Here's the drawing with two shaded views (mm, measured from the low corner). I have some questions. A direction names the side the tool comes from. Coordinates: 2 decimals unless noted, no trailing zeros. Write each loop counter-clockwise with the first axis right and the second up, starting at its lowest first coordinate (ties: lowest second). Pieces come first, ordered by that corner, then holes.
Item 1: For P1, Ø7, axis at x = 21, y = 12, coming from the -Z side; P2, Ø0.6, axis at y = 1, z = 0.5, coming from the -X side; P3, Ø0.6, axis at y = 0.5, z = 0.5, coming from the +X side; P4, Ø4, axis at x = 39, y = 17, coming from the +Z side, each with a flat end and sliding along its axis, tell me the tip position at first contact or that it passes through.
Item 2: I want a section at D-D on z = 0.6. Please give me the cut outline in (x, y).
Item 3: If I drill on probe 1 along Y at (x, z) = (4, 0.8) (1 decimal); probe 2 along X at (y, z) = (16.5, 0.45) (1 decimal); probe 3 along X at (y, z) = (17.5, 1.5) (1 decimal), over which ranges is the centre line in solid material (lowest first)?
Item 4: I want a section at B-B on y = 10.25. Please give me the cut outline in (x, z).
Item 5: I want a section at A-A on x = 39. Please give me the cut outline in (y, z), then the cut area to 3 significant figures.
Item 6: I want a section at C-C on x = 22.5. Please give me the cut outline in (y, z) (1 decimal).
Item 7: Which directions (+Z, -Z, +X, -X, +Y, -Y) give clear straight access to the entire face, cutting with the end or side of a thin tool? Please do the marked faces 1 and 2.
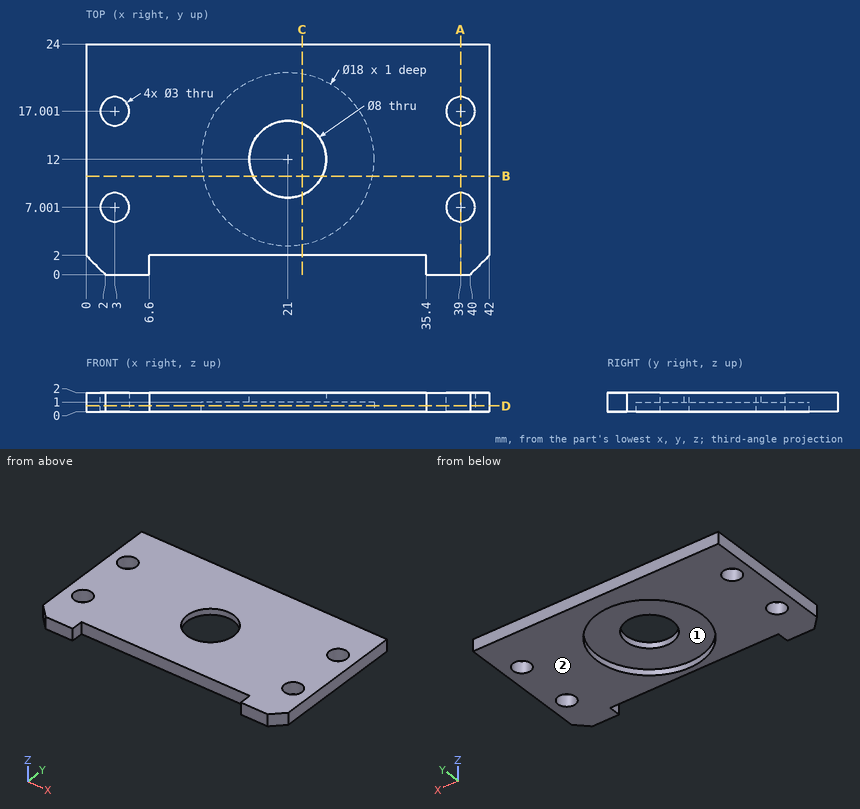
Response values:
1. P1: passes through
1. P2: stops at x = 0.7
1. P3: stops at x = 40.8
1. P4: stops at z = 2
2. outline: (0, 2) - (2, 0) - (6.6, 0) - (6.6, 2) - (35.4, 2) - (35.4, 0) - (40, 0) - (42, 2) - (42, 24) - (0, 24) - close; hole circle Ø3 at (3, 7); hole circle Ø3 at (3, 17); hole circle Ø18 at (21, 12); hole circle Ø3 at (39, 7); hole circle Ø3 at (39, 17)
3. probe 1: y = 0 to 5.9, 8.1 to 15.9, 18.1 to 24
3. probe 2: x = 0 to 1.6, 4.4 to 13.2, 28.8 to 37.6, 40.4 to 42
3. probe 3: x = 0 to 1.6, 4.4 to 37.6, 40.4 to 42
4. outline: (0, 0) - (12.17, 0) - (12.17, 1) - (17.4, 1) - (17.4, 2) - (0, 2) - close; (24.6, 1) - (29.83, 1) - (29.83, 0) - (42, 0) - (42, 2) - (24.6, 2) - close
5. outline: (0, 0) - (5.5, 0) - (5.5, 2) - (0, 2) - close; (8.5, 0) - (15.5, 0) - (15.5, 2) - (8.5, 2) - close; (18.5, 0) - (24, 0) - (24, 2) - (18.5, 2) - close
5. area: 36.0 mm2
6. outline: (2, 0) - (3.1, 0) - (3.1, 1) - (8.3, 1) - (8.3, 2) - (2, 2) - close; (15.7, 1) - (20.9, 1) - (20.9, 0) - (24, 0) - (24, 2) - (15.7, 2) - close
7. face 1: -Z
7. face 2: -Z, +X, -X, +Y, -Y
